Geometry check sheet. Reference: the model listing, model coordinates, mm. A direction names the side the tool comes from. Round coordinates to 2 decimals unless told otherwise and drop trailing zeros. Write each loop counter-clockwise with the first axis right and the second up, starting at its lowest first coordinate (ties: lowest second). Pieces come first, ordered by that corner, then holes. Notation, with made-up numbers: (-6.5, 18.5) -> (6.5, 18.5) arc R21 ccw to (6.5, 32.5) -> close; hole circle Ø8 at (37, 24.5). An arc over 180 degrees is marked (long way). Use a Markdown table: item, result.
```python
from build123d import *

# Parameters (mm, degrees)
SKETCH_1_R      = 4
EXTRUDE_1_DEPTH = 24
SKETCH_2_R      = 3
EXTRUDE_2_DEPTH = 23
EXTRUDE_START   = 66
SKETCH_3_R      = 3
EXTRUDE_3_DEPTH = 66
SKETCH_4_R      = 2.5
EXTRUDE_4_DEPTH = 5
EXTRUDE_START_2 = 5
SKETCH_6_R      = 2.5
EXTRUDE_5_DEPTH = 5


with BuildPart() as part:
    # 草图1 → 凸台-拉伸1 (new body)
    with BuildSketch(Plane.XY):
        Circle(SKETCH_1_R)
    extrude(amount=EXTRUDE_1_DEPTH)

    # 草图2 → 凸台-拉伸2 (add)
    with BuildSketch(Plane.XY.offset(24)):
        Circle(SKETCH_2_R)
    extrude(amount=EXTRUDE_2_DEPTH)

    # 草图3 → 凸台-拉伸3 (add)
    with BuildSketch(Plane(origin=(0, 0, 0), x_dir=(-1, 0, 0), z_dir=(0, 0, -1)).offset(EXTRUDE_START)):
        with Locations(Location((0, 0, 0), (0, 0, 180))):
            Circle(SKETCH_3_R)
    extrude(amount=-EXTRUDE_3_DEPTH)

    # 草图4 → 凸台-拉伸4 (add)
    with BuildSketch(Plane(origin=(0, 0, -66), x_dir=(-1, 0, 0), z_dir=(0, 0, -1))):
        Circle(SKETCH_4_R)
    extrude(amount=EXTRUDE_4_DEPTH)

    # 草图6 → 凸台-拉伸5 (add)
    with BuildSketch(Plane.XY.offset(47).offset(EXTRUDE_START_2)):
        with Locations(Location((0, 0, 0), (0, 0, 180))):
            Circle(SKETCH_6_R)
    extrude(amount=-EXTRUDE_5_DEPTH)


solid = part.part
```
(1) Gauge pin test, flat ends, axial feed: pin 1 Ø1 at (x, y) = (2.5, -3) entering from +Z; pin 2 Ø2 at (x, z) = (-0.5, -14) entering from -Y; pin 3 Ø2 at (x, z) = (-3, 34) entering from +Y. Record the tip position at first contact, or that the pin passes through.
A:
| item | result |
|---|---|
| pin 1 | stops at z = 24 |
| pin 2 | stops at y = -3 |
| pin 3 | stops at y = 2.24 |
(2) Section check B-B on z = 44. Record the cut outline in (x, y).
A:
| item | result |
|---|---|
| outline | circle Ø6 at (0, 0) |
(3) Access from +Z, -Z, +X, -X, +Y, -Y to the whole of each face (thin tool, end or side, straight path). Record for faces 1 (the face through (1, 3, 24)), 2 (the face through (1, 3, 0)), 3 (the face through (0, 0, 52)).
A:
| item | result |
|---|---|
| face 1 | +Z |
| face 2 | -Z |
| face 3 | +Z, +X, -X, +Y, -Y |
(4) Thickness scan on line 1 (Z direction, x = -1.75, y = -2.75); line 2 (Y direction, x = 0.25, z = 34); line 3 (Y direction, x = -1.5, z = 27). Record the ranges inside material, lowest first.
A:
| item | result |
|---|---|
| line 1 | z = 0 to 24 |
| line 2 | y = -2.99 to 2.99 |
| line 3 | y = -2.6 to 2.6 |
(5) Section check A-A on x = 0. Record the cut outline in (y, z), plus the area to 3 significant figures.
A:
| item | result |
|---|---|
| outline | (-4, 0) -> (-3, 0) -> (-3, -66) -> (-2.5, -66) -> (-2.5, -71) -> (2.5, -71) -> (2.5, -66) -> (3, -66) -> (3, 0) -> (4, 0) -> (4, 24) -> (3, 24) -> (3, 47) -> (2.5, 47) -> (2.5, 52) -> (-2.5, 52) -> (-2.5, 47) -> (-3, 47) -> (-3, 24) -> (-4, 24) -> close |
| area | 776 mm2 |
